from build123d import *
from build123d.topology import SkipClean

# Parameters (mm, degrees)
BOSS_EXTRUDE1_DEPTH      = 1
BOSS_EXTRUDE2_DEPTH      = 18
BOSS_EXTRUDE2_DEPTH_BACK = 18.972201
SKETCH2_W                = 8
SKETCH2_H                = 7.75
SKETCH3_R                = 59.910539196
CUT_EXTRUDE1_DEPTH       = 28.577289765
CUT_EXTRUDE2_DEPTH       = 28.577289597
CUT_EXTRUDE2_DEPTH_BACK  = 28.577289597
SKETCH5_R                = 1.4
BOSS_EXTRUDE3_DEPTH      = 8.75
CUT_EXTRUDE3_DEPTH       = 28.276489905
FILLET1_R                = 2
FILLET2_R                = 0.5


with BuildPart() as part:
    # Sketch1 → Boss-Extrude1 (new body)
    with BuildSketch(Plane(origin=(0, 0, 0), x_dir=(1, 0, 0), z_dir=(0, 1, 0))):
        with BuildLine():
            Line((-1, 17.972200756), (-1, 18.972200756))
            Line((-1, 18.972200756), (1, 18.972200756))
            Line((1, 18.972200756), (1, 17.972200756))
            ThreePointArc((1, 17.972200756), (0, -18), (-1, 17.972200756))
        make_face()
    extrude(amount=BOSS_EXTRUDE1_DEPTH)

    # Sketch2 → Boss-Extrude2 (add, two sides: drawn at the far end of the back side and taken through both)
    with BuildSketch(Plane.XY.offset(-BOSS_EXTRUDE2_DEPTH_BACK)):
        with Locations((-12.05, 4.875)):
            Rectangle(SKETCH2_W, SKETCH2_H)
        with Locations((12.05, 4.875)):
            Rectangle(SKETCH2_W, SKETCH2_H)
    extrude(amount=BOSS_EXTRUDE2_DEPTH + BOSS_EXTRUDE2_DEPTH_BACK)

    # Sketch3 → Cut-Extrude1 (cut, through all)
    with BuildSketch(Plane.XZ):
        Circle(SKETCH3_R)
        with BuildLine():
            Line((-1, -17.972200756), (-1, -18.972200756))
            Line((-1, -18.972200756), (1, -18.972200756))
            Line((1, -18.972200756), (1, -17.972200756))
            ThreePointArc((1, -17.972200756), (0, 18), (-1, -17.972200756))
        make_face(mode=Mode.SUBTRACT)
    extrude(amount=-CUT_EXTRUDE1_DEPTH, mode=Mode.SUBTRACT)

    # Sketch5 → Cut-Extrude2 (cut, two sides: drawn at the far end of the back side and taken through both)
    with BuildSketch(Plane(origin=(0, 0, 0), x_dir=(1, 0, 0), z_dir=(0, 1, 0)).offset(-CUT_EXTRUDE2_DEPTH_BACK)):
        with Locations(Location((0, 0, 0), (0, 0, 180))):
            Circle(SKETCH5_R)
        with Locations(Location((11, -4, 0), (0, 0, 180))):
            Circle(SKETCH5_R)
        with Locations(Location((-11, -4, 0), (0, 0, 180))):
            Circle(SKETCH5_R)
        with Locations(Location((-11.691342951, 6.75, 0), (0, 0, 180))):
            Circle(SKETCH5_R)
        with Locations(Location((0, -13.5, 0), (0, 0, 180))):
            Circle(SKETCH5_R)
        with Locations(Location((11.691342951, 6.75, 0), (0, 0, 180))):
            Circle(SKETCH5_R)
    extrude(amount=CUT_EXTRUDE2_DEPTH + CUT_EXTRUDE2_DEPTH_BACK, mode=Mode.SUBTRACT)

    # Sketch6 → Boss-Extrude3 (add)
    with SkipClean():  # the faces are left unmerged after this step: merging them gives an invalid solid
        with BuildSketch(Plane.XZ):
            with BuildLine():
                Line((-8.097530488, -15.075758147), (8.097530488, -15.075758147))
                Line((8.097530488, -15.075758147), (8.097530488, -16.075758147))
                ThreePointArc((8.097530488, -16.075758147), (4.646545909, -17.389928439), (1, -17.972200756))
                Line((1, -17.972200756), (1, -18.972200756))
                Line((1, -18.972200756), (-1, -18.972200756))
                Line((-1, -18.972200756), (-1, -17.972200756))
                ThreePointArc((-1, -17.972200756), (-4.646545909, -17.389928439), (-8.097530488, -16.075758147))
                Line((-8.097530488, -16.075758147), (-8.097530488, -15.075758147))
            make_face()
        extrude(amount=-BOSS_EXTRUDE3_DEPTH)
    add(part.part.scale(1), mode=Mode.REPLACE)  # the faces are merged on a copy

    # Sketch7 → Cut-Extrude3 (cut, through all)
    with BuildSketch(Plane(origin=(0, 1, 0), x_dir=(1, 0, 0), z_dir=(0, 1, 0))):
        with BuildLine():
            Line((16.05, 8.148466113), (16.05, -8.148466113))
            ThreePointArc((16.05, -8.148466113), (18, 0), (16.05, 8.148466113))
        make_face()
        with BuildLine():
            Line((-16.05, -8.148466113), (-16.05, 8.148466113))
            ThreePointArc((-16.05, 8.148466113), (-18, 0), (-16.05, -8.148466113))
        make_face()
    extrude(amount=-CUT_EXTRUDE3_DEPTH, mode=Mode.SUBTRACT)

    # Fillet1
    # the kernel refuses this fillet: 2 mm, written as the material it takes off along each edge
    with BuildSketch(Plane(origin=(16.05, 0, 13.148466113), x_dir=(-1, 0, 0), z_dir=(0, 0, -1)), Plane(origin=(-16.05, 0, -13.148466113), x_dir=(1, 0, 0), z_dir=(0, 0, 1))) as fillet1_piece_1:
        with BuildLine():
            CenterArc((FILLET1_R, FILLET1_R), FILLET1_R, 180, 90)
            Line((0, FILLET1_R), (0, 0))
            Line((0, 0), (FILLET1_R, 0))
        make_face()
    extrude(amount=26.296932227, mode=Mode.SUBTRACT)
    with BuildSketch(Plane(origin=(0, 0, 0), x_dir=(0.9816654427410076, 0, 0.19061206291339847), z_dir=(0.19061206291339847, 0, -0.9816654427410076))) as fillet1_piece_2:
        with BuildLine():
            CenterArc((18 - FILLET1_R, -FILLET1_R), FILLET1_R, 0, 90)
            Line((18, -FILLET1_R), (18, 0))
            Line((18, 0), (18 - FILLET1_R, 0))
        make_face()
    revolve(axis=Axis((0, 0, 0), (0, -1, 0)), revolution_arc=158.022988726, mode=Mode.SUBTRACT)
    with BuildSketch(Plane(origin=(0, 0, 0), x_dir=(0.4498628048748618, 0, -0.8930976748318865), z_dir=(-0.8930976748318865, 0, -0.4498628048748618))) as fillet1_piece_3:
        with BuildLine():
            CenterArc((18 - FILLET1_R, -FILLET1_R), FILLET1_R, 0, 90)
            Line((18, -FILLET1_R), (18, 0))
            Line((18, 0), (18 - FILLET1_R, 0))
        make_face()
    revolve(axis=Axis((0, 0, 0), (0, -1, 0)), revolution_arc=52.265087313, mode=Mode.SUBTRACT)
    with BuildSketch(Plane(origin=(0, 0, 0), x_dir=(-0.9816270812345659, 0, -0.19080952121659656), z_dir=(-0.19080952121659656, 0, 0.9816270812345659))) as fillet1_piece_4:
        with BuildLine():
            CenterArc((18 - FILLET1_R, -FILLET1_R), FILLET1_R, 0, 90)
            Line((18 - FILLET1_R, 0), (18, 0))
            Line((18, 0), (18, -FILLET1_R))
        make_face()
    revolve(axis=Axis((0, 0, 0), (0, -1, 0)), revolution_arc=52.265087313, mode=Mode.SUBTRACT)
    with BuildSketch(Plane(origin=(0, 0, 0), x_dir=(-0.44986280487485913, 0, -0.8930976748318878), z_dir=(-0.8930976748318878, 0, 0.44986280487485913))) as fillet1_piece_5_section:
        with BuildLine():
            CenterArc((18 - FILLET1_R, -FILLET1_R), FILLET1_R, 0, 90)
            Line((18 - FILLET1_R, 0), (18, 0))
            Line((18, 0), (18, -FILLET1_R))
        make_face()
    fillet1_piece_5 = revolve(axis=Axis((0, 0, 0), (0, -1, 0)), revolution_arc=39.46607541, mode=Mode.PRIVATE)
    fillet1_piece_5 = split(fillet1_piece_5, bisect_by=Plane(origin=(-1, 0.459921415, -16.842636156), z_dir=(-1, 0, 0)), keep=Keep.TOP, mode=Mode.PRIVATE)
    add(fillet1_piece_5, mode=Mode.SUBTRACT)
    with BuildSketch(Plane(origin=(0, 0, 0), x_dir=(-0.44986280487485913, 0, -0.8930976748318878), z_dir=(-0.8930976748318878, 0, 0.44986280487485913))) as fillet1_piece_6_section:
        with BuildLine():
            CenterArc((18 - FILLET1_R, -FILLET1_R), FILLET1_R, 0, 90)
            Line((18 - FILLET1_R, 0), (18, 0))
            Line((18, 0), (18, -FILLET1_R))
        make_face()
    fillet1_piece_6 = revolve(axis=Axis((0, 0, 0), (0, -1, 0)), revolution_arc=39.46607541, mode=Mode.PRIVATE)
    fillet1_piece_6 = split(fillet1_piece_6, bisect_by=Plane(origin=(1, 0.461212135, -17.370872929), z_dir=(1, 0, 0)), keep=Keep.TOP, mode=Mode.PRIVATE)
    add(fillet1_piece_6, mode=Mode.SUBTRACT)
    with BuildSketch(Plane(origin=(0, 0, 0), x_dir=(-0.22037727986092012, 0, -0.9754147089936167), z_dir=(-0.9754147089936167, 0, 0.22037727986092012))) as fillet1_piece_7_section:
        with BuildLine():
            CenterArc((18 - FILLET1_R, -FILLET1_R), FILLET1_R, 0, 90)
            Line((18, -FILLET1_R), (18, 0))
            Line((18, 0), (18 - FILLET1_R, 0))
        make_face()
    fillet1_piece_7 = revolve(axis=Axis((0, 0, 0), (0, -1, 0)), revolution_arc=39.46607541, mode=Mode.PRIVATE)
    fillet1_piece_7 = split(fillet1_piece_7, bisect_by=Plane(origin=(-1, 0.461212076, -17.370872697), z_dir=(-1, 0, 0)), keep=Keep.TOP, mode=Mode.PRIVATE)
    add(fillet1_piece_7, mode=Mode.SUBTRACT)
    with BuildSketch(Plane(origin=(0, 0, 0), x_dir=(-0.22037727986092012, 0, -0.9754147089936167), z_dir=(-0.9754147089936167, 0, 0.22037727986092012))) as fillet1_piece_8_section:
        with BuildLine():
            CenterArc((18 - FILLET1_R, -FILLET1_R), FILLET1_R, 0, 90)
            Line((18, -FILLET1_R), (18, 0))
            Line((18, 0), (18 - FILLET1_R, 0))
        make_face()
    fillet1_piece_8 = revolve(axis=Axis((0, 0, 0), (0, -1, 0)), revolution_arc=39.46607541, mode=Mode.PRIVATE)
    fillet1_piece_8 = split(fillet1_piece_8, bisect_by=Plane(origin=(1, 0.459921447, -16.842636316), z_dir=(1, 0, 0)), keep=Keep.TOP, mode=Mode.PRIVATE)
    add(fillet1_piece_8, mode=Mode.SUBTRACT)

    # Fillet2
    fillet2_edges = [part.edges().sort_by_distance(p)[0] for p in [
        (16.05, 8.75, 0),
        (-16.05, 8.75, 0),
        (-12.688880148, 8.75, 12.766844582),
        (-12.707725875, 8.75, -12.748086252),
        (12.688880148, 8.75, 12.766844582),
        (12.707725875, 8.75, -12.748086252),
    ]]
    fillet(fillet2_edges, radius=FILLET2_R)


solid = part.part
Could you check a few things on this model? Use its own coordinates, in mm. A direction names the side the tool comes from. Coordinates: 2 decimals unless noted, no trailing zeros. Write each loop counter-clockwise with the first axis right and the second up, starting at its lowest first coordinate (ties: lowest second). Pieces come first, ordered by that corner, then holes. Notation, with made-up numbers: (20, -29.75) - (73, -29.75) arc R20 cw to (73, -5.75) - close; hole circle Ø11 at (15, 6). An arc over 180 degrees is marked (long way). Write item = value, one per line.
1) Please list where these lines run through material, in increasing order: line 1 (X direction, y = 5.5, z = 4); line 2 (X direction, y = 4, z = -6.75); line 3 (Y direction, x = 8, z = -8). Write a range as [from, to].
Result set:
line_1 = [-16.05, -12.4], [-9.6, -8.05], [8.05, 9.6], [12.4, 16.05]
line_2 = [-16.05, -13.09], [-10.29, -8.05], [8.05, 10.29], [13.09, 16.05]
line_3 = [0, 1]
2) Suppose I cut it at B-B on x = 0. Please give me the cut outline in (y, z), plus the area to 3 significant figures.
Result set:
outline = (0, -18.97) - (8.75, -18.97) - (8.75, -15.08) - (1, -15.08) - (1, -1.4) - (0, -1.4) - close; (0, 1.4) - (1, 1.4) - (1, 12.1) - (0, 12.1) - close; (0, 14.9) - (1, 14.9) - (1, 17.73) arc R2 ccw to (0, 16) - close
area = 60.8 mm2
3) Will these pins go through, and if not, where does the flat tip stop? pin 1 Ø3.5 at (x, z) = (0, 0) entering from +Y; pin 2 Ø2.5 at (x, z) = (0, 13.5) entering from -Y; pin 3 Ø8 at (x, z) = (10, 7.5) entering from -Y; pin 4 Ø2.5 at (y, z) = (5, -17) entering from -X.
Result set:
pin_1 = 1
pin_2 = through
pin_3 = 0
pin_4 = -8.71
4) Suppose I cut it at D-D on y = 2.5. Please give me the cut outline in (x, z), plus the area to 3 significant figures.
Result set:
outline = (-16.05, -8.15) arc R18 ccw to (-1, -17.97) - (-1, -18.97) - (1, -18.97) - (1, -17.97) arc R18 ccw to (16.05, -8.15) - (16.05, 8.15) arc R18 ccw to (8.05, 16.1) - (8.05, -15.08) - (-8.05, -15.08) - (-8.05, 16.1) arc R18 ccw to (-16.05, 8.15) - close; hole circle Ø2.8 at (-11.69, -6.75); hole circle Ø2.8 at (-11, 4); hole circle Ø2.8 at (11, 4); hole circle Ø2.8 at (11.69, -6.75)
area = 430 mm2
5) For faces 4 (the cylindrical face through (1.4, 0.49, 0.06)), 5 (the flat face through (-2, 1, 1)), which set-ups out of +Z, -Z, +X, -X, +Y, -Y let a thin tool reach every point of the face, with its end or its side?
Result set:
face_4 = +Y, -Y
face_5 = +Z, +Y
6) We'd pull the mould along Z, two halves only. Please class faces 1 (the cylindrical face through (9.728, 5.081, -15.145)), 2 (the flat face through (0, 0, -2)), 3 (the cylindrical face through (12.4, 4.31, 4.06)): +Z half, -Z half, draft (parallel to the pull), parting line (faces both ways), or undercut.
Result set:
face_1 = -Z half
face_2 = draft
face_3 = undercut
7) Suppose I cut it at C-C on z = 0. Please give me the cut outline in (x, y).
Result set:
outline = (-16.05, 2) arc R2 ccw to (-14.05, 0) - (-1.4, 0) - (-1.4, 1) - (-8.05, 1) - (-8.05, 8.75) - (-15.55, 8.75) arc R0.5 ccw to (-16.05, 8.25) - close; (1.4, 0) - (14.05, 0) arc R2 ccw to (16.05, 2) - (16.05, 8.25) arc R0.5 ccw to (15.55, 8.75) - (8.05, 8.75) - (8.05, 1) - (1.4, 1) - close
8) Suppose I cut it at A-A on z = -6.75. Please give me the cut outline in (x, y), plus the area to 3 significant figures.
Result set:
outline = (-16.05, 2) arc R2 ccw to (-14.05, 0) - (-13.09, 0) - (-13.09, 8.75) - (-15.55, 8.75) arc R0.5 ccw to (-16.05, 8.25) - close; (-10.29, 0) - (10.29, 0) - (10.29, 8.75) - (8.05, 8.75) - (8.05, 1) - (-8.05, 1) - (-8.05, 8.75) - (-10.29, 8.75) - close; (13.09, 0) - (14.05, 0) arc R2 ccw to (16.05, 2) - (16.05, 8.25) arc R0.5 ccw to (15.55, 8.75) - (13.09, 8.75) - close
area = 105 mm2
